Geometry check sheet. Reference: the model listing, model coordinates, mm. A direction names the side the tool comes from. Give positions to 0.01 mm unless a question says otherwise; leave off trailing zeros. Loops run counter-clockwise (first coordinate to the right, second up) from the corner with the lowest first, then second, coordinate; pieces in that order, holes last.
1. Go/stop test with flat-tipped pins: pin 1 Ø1.7 at (y, z) = (7, 3.5) entering from +X; pin 2 Ø1.7 at (y, z) = (6, 3.5) entering from -X; pin 3 Ø2.5 at (y, z) = (6, 3) entering from +X. Record where each tip stops, or that it passes through.
2. Cross-section at D-D, the plane z = 1.8. Record the cut outline in (x, y), plus the area to 3 significant figures.
3. Release check for a two-part mould opening along X. For faces 1 (the flat face through (-4, 4.286, 3)), 2 (the flat face through (4, -7.143, 3)), 3 (the flat face through (-1.429, -9, 3)) record: +X half, -X half, draft (parallel to the pull), parting line (faces both ways), or undercut.
4. Cross-section at B-B, the plane x = -2.5. Record the cut outline in (y, z).
5. Tool access check on faces 4 (the flat face through (-4, -7.143, 3)), 5 (the flat face through (4, 7, 2.143)), 6 (the flat face through (-4, 1.429, 3)). Record the directions out of +Z, -Z, +X, -X, +Y, -Y that give a thin tool (end or side, any length) a straight path to the whole face; none if there is none.
6. Cross-section at A-A, the plane z = 3.15. Record the cut outline in (x, y), plus the area to 3 significant figures.
7. Material ranges on L1, parallel to Y at x = -1.5, z = 2.25; L2, parallel to Z at x = 4.5, y = 8; L3, parallel to X at y = -9, z = 3.5, recorded low to high.
8. Cross-section at C-C, the plane y = -1. Record the cut outline in (x, z), plus the area to 3 significant figures.
from build123d import *

# Parameters (mm, degrees)
F0_R     = 14
F1_DEPTH = 3
F2_W     = 8
F2_H     = 8
F3_DEPTH = 3
F4_SCALE = 0.7143


with BuildPart() as f1:
    # F0 (on Top) → F1 (new body)
    with BuildSketch(Plane.XY):
        Circle(F0_R)
    extrude(amount=F1_DEPTH)

    # F2 (on face) → F3 (join)
    with BuildSketch(Plane.XY.offset(3)):
        with BuildLine():
            Line((-10, 6), (-10, 9.7979589711))
            ThreePointArc((-10, 9.7979589711), (-12.9614813968, 5.2915026221), (-14, 0))
            ThreePointArc((-14, 0), (-12.9068087767, -5.4234940031), (-9.7979589711, -10))
            Line((-9.7979589711, -10), (-2, -10))
            Line((-2, -10), (-2, -13.8564064606))
            ThreePointArc((-2, -13.8564064606), (0, -14), (2, -13.8564064606))
            Line((2, -13.8564064606), (2, -10))
            Line((2, -10), (9.7979589711, -10))
            ThreePointArc((9.7979589711, -10), (12.9068087767, -5.4234940031), (14, 0))
            ThreePointArc((14, 0), (12.9614813968, 5.2915026221), (10, 9.7979589711))
            Line((10, 9.7979589711), (10, 6))
            Line((10, 6), (2, 6))
            Line((2, 6), (2, 13.8564064606))
            ThreePointArc((2, 13.8564064606), (0, 14), (-2, 13.8564064606))
            Line((-2, 13.8564064606), (-2, 6))
            Line((-2, 6), (-10, 6))
        make_face()
        with Locations((-6, -2)):
            Rectangle(F2_W, F2_H, mode=Mode.SUBTRACT)
        with Locations((6, -2)):
            Rectangle(F2_W, F2_H, mode=Mode.SUBTRACT)
    extrude(amount=F3_DEPTH)


with BuildPart() as f1_1:
    # F4: moved
    add(f1.part.scale(F4_SCALE))


solid = f1_1.part
Result:
1. pin 1: stops at x = 7.89
1. pin 2: stops at x = -8.57
1. pin 3: stops at x = 8.8
2. outline: circle Ø20 at (0, 0)
2. area: 314 mm2
3. face 1: undercut
3. face 2: draft
3. face 3: -X half
4. outline: (-9.68, 0) - (9.68, 0) - (9.68, 2.14) - (4.29, 2.14) - (4.29, 4.29) - (1.43, 4.29) - (1.43, 2.14) - (-4.29, 2.14) - (-4.29, 4.29) - (-7.14, 4.29) - (-7.14, 2.14) - (-9.68, 2.14) - close
5. face 4: +Z, -X, -Y
5. face 5: +Z, +Y
5. face 6: +Z
6. outline: (-7.14, 4.29) - (-7.14, 7) arc R10 ccw to (-7, -7.14) - (-1.43, -7.14) - (-1.43, -9.9) arc R10 ccw to (1.43, -9.9) - (1.43, -7.14) - (7, -7.14) arc R10 ccw to (7.14, 7) - (7.14, 4.29) - (1.43, 4.29) - (1.43, 9.9) arc R10 ccw to (-1.43, 9.9) - (-1.43, 4.29) - close; hole (-7.14, -4.29) - (-1.43, -4.29) - (-1.43, 1.43) - (-7.14, 1.43) - close; hole (1.43, -4.29) - (7.14, -4.29) - (7.14, 1.43) - (1.43, 1.43) - close
6. area: 177 mm2
7. L1: y = -7.14 to -4.29, 1.43 to 4.29
7. L2: z = 0 to 2.14
7. L3: x = -1.43 to 1.43
8. outline: (-9.95, 0) - (9.95, 0) - (9.95, 4.29) - (7.14, 4.29) - (7.14, 2.14) - (1.43, 2.14) - (1.43, 4.29) - (-1.43, 4.29) - (-1.43, 2.14) - (-7.14, 2.14) - (-7.14, 4.29) - (-9.95, 4.29) - close
8. area: 60.8 mm2
